Check sheet for the drawn part. Datum: minimum x, y, z corner. Units: mm. Give positions to 0.01 mm unless a question says otherwise; leave off trailing zeros. Order: outer loops, then holes, each group sorted by start corner. A loop starts at its lowest first (then second) coordinate and runs counter-clockwise, first axis right, second up. Notation, with made-up numbers: M 47.5,46.5 L 80.5,46.5 A25 ccw 80.5,70.5 Z; hole C -11.5,-21.75 d6. An arc over 180 degrees is marked long. Answer as CSV lines item,"result". Start each with the question number.
Q1. Section check A-A, the plane z = 2.65. Record the boundary of the cut face in (x, y).
Q2. Go/stop test with a flat-tipped pin: pin 1 (1.4 mm diameter, centred on x = 2.5, y = 2, fed in from -Z). Record where the tip stops, or that it passes through.
Q3. Thickness scan on line 1 (Y direction, x = 2.5, z = 0.75); line 2 (X direction, y = 2, z = 2.4); line 3 (Y direction, x = 17.5, z = 2.45). Record the ranges inside material, lowest first.
Q4. Section check D-D, the plane z = 1.3. Record the boundary of the cut face in (x, y), then the cut area to 3 significant figures.
Q5. Section check C-C, the plane x = 2.5. Record the boundary of the cut face in (y, z), then the cut area to 3 significant figures.
Q6. Mould release check, pull along X, two halves, no side actions. Record for the marked faces 1, 2, 3 and 4: +X half, -X half, draft (parallel to the pull), parting line (faces both ways), or undercut.
Q7. Section check B-B, the plane y = 13. Record the boundary of the cut face in (x, z), then the cut area to 3 significant figures.
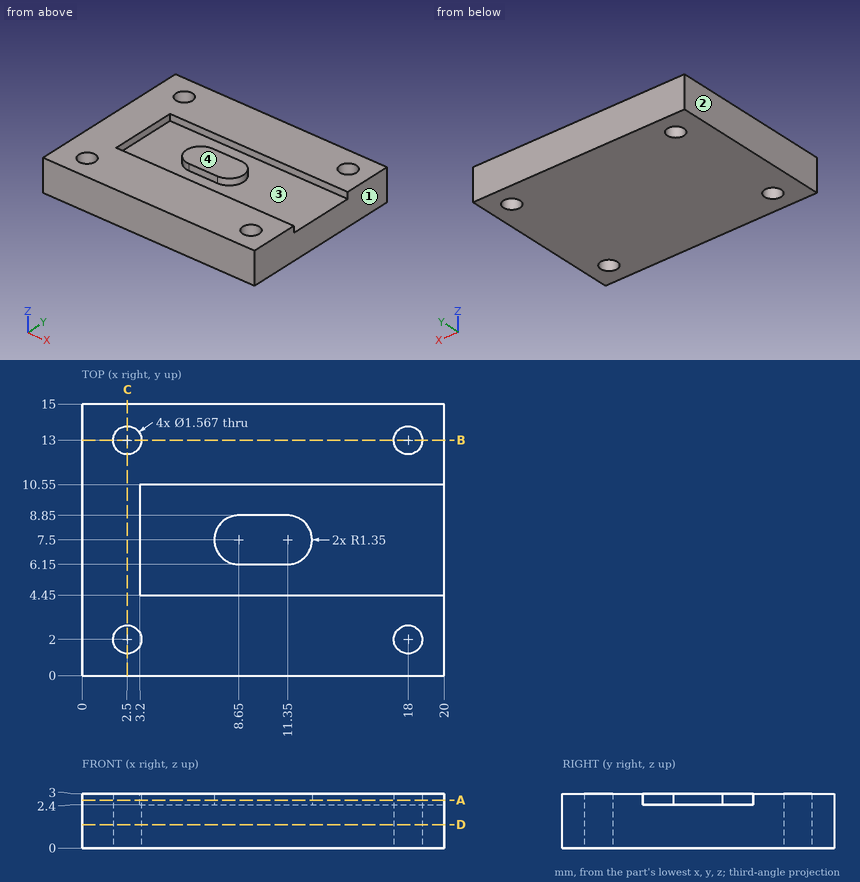
Answer block:
1,outline,"M 0,0 L 20,0 L 20,4.45 L 3.2,4.45 L 3.2,10.55 L 20,10.55 L 20,15 L 0,15 Z; M 8.65,6.15 L 11.35,6.15 A1.35 ccw 11.35,8.85 L 8.65,8.85 A1.35 ccw Z; hole C 2.5,2 d1.57; hole C 2.5,13 d1.57; hole C 18,2 d1.57; hole C 18,13 d1.57"
2,pin 1,"passes through"
3,line 1,"y = 0 to 1.22, 2.78 to 12.22, 13.78 to 15"
3,line 2,"x = 0 to 1.72, 3.28 to 17.22, 18.78 to 20"
3,line 3,"y = 0 to 1.4, 2.6 to 4.45, 10.55 to 12.4, 13.6 to 15"
4,outline,"M 0,0 L 20,0 L 20,15 L 0,15 Z; hole C 2.5,2 d1.57; hole C 2.5,13 d1.57; hole C 18,2 d1.57; hole C 18,13 d1.57"
4,area,"292 mm2"
5,outline,"M 0,0 L 1.22,0 L 1.22,3 L 0,3 Z; M 2.78,0 L 12.22,0 L 12.22,3 L 2.78,3 Z; M 13.78,0 L 15,0 L 15,3 L 13.78,3 Z"
5,area,"35.6 mm2"
6,face 1,"+X half"
6,face 2,"-X half"
6,face 3,"undercut"
6,face 4,"draft"
7,outline,"M 0,0 L 1.72,0 L 1.72,3 L 0,3 Z; M 3.28,0 L 17.22,0 L 17.22,3 L 3.28,3 Z; M 18.78,0 L 20,0 L 20,3 L 18.78,3 Z"
7,area,"50.6 mm2"
